from build123d import *

# Parameters (mm, degrees)
BOSS_EXTRUDE1_DEPTH = 9
SKETCH2_R           = 2.875
BOSS_EXTRUDE2_DEPTH = 7
SKETCH3_W           = 1.5
SKETCH3_H           = 1.5
BOSS_EXTRUDE3_DEPTH = 6


with BuildPart() as part:
    # Sketch1 → Boss-Extrude1 (new body)
    with BuildSketch(Plane.XY):
        Polygon((3.4, 0), (1.7, 2.944486373), (-1.7, 2.944486373), (-3.4, 0), (-1.7, -2.944486373), (1.7, -2.944486373), align=None)
    extrude(amount=BOSS_EXTRUDE1_DEPTH)

    # Sketch2 → Boss-Extrude2 (add)
    with BuildSketch(Plane.XY.offset(9)):
        Circle(SKETCH2_R)
    extrude(amount=BOSS_EXTRUDE2_DEPTH)

    # Sketch3 → Boss-Extrude3 (add)
    with BuildSketch(Plane.XY.offset(16)):
        with Locations((0, 2.875)):
            Rectangle(SKETCH3_W, SKETCH3_H)
    extrude(amount=-BOSS_EXTRUDE3_DEPTH)


solid = part.part
Geometry: final body of the model. Coordinates: model frame, mm. A direction names the side the tool comes from. Round coordinates to 2 decimals unless told otherwise and drop trailing zeros. Loops run counter-clockwise (first coordinate to the right, second up) from the corner with the lowest first, then second, coordinate; pieces in that order, holes last.
Q1. Section D-D on y = -2. Return loops of the section in (x, z), plus the area to 3 significant figures.
Q2. Material intervals for L1, parallel to Z at x = 2, y = 2.25; L2, parallel to Y at x = -1.25, z = 6.75; L3, parallel to X at y = -2, z = 13.75, sorted ascending.
Q3. Section B-B on z = 2. Return loops of the section in (x, y).
Q4. Pin query (flat end, axial travel): P1, Ø1.5, axis at x = -0.5, z = 2, coming from the +Y side; P2, Ø2, axis at x = -1, z = 11.5, coming from the -Y side (3 decimals). Return the tip coordinate at first contact, or that it passes through.
Q5. Access query for faces 1 (the flat face through (0.75, 3, 13)), 2 (the flat face through (0, 2.944, 4)), 3 (the flat face through (-0.75, 3, 13)). Directions: +Z, -Z, +X, -X, +Y, -Y. A direction counts if a zero-diameter tool reaches every point of the face in a straight line with its end or side. Return the directions, or none.
Q6. Section A-A on x = 0. Return loops of the section in (y, z) (3 decimals).
Q7. Section C-C on y = 1.5. Return loops of the section in (x, z).
Evaluation:
1. outline: (-2.25, 0) - (2.25, 0) - (2.25, 9) - (2.07, 9) - (2.07, 16) - (-2.07, 16) - (-2.07, 9) - (-2.25, 9) - close
1. area: 69.3 mm2
2. L1: z = 0 to 9
2. L2: y = -2.94 to 2.94
2. L3: x = -2.07 to 2.07
3. outline: (-3.4, 0) - (-1.7, -2.94) - (1.7, -2.94) - (3.4, 0) - (1.7, 2.94) - (-1.7, 2.94) - close
4. P1: stops at y = 2.94
4. P2: stops at y = -2.875
5. face 1: +Z, +X, +Y
5. face 2: -Z, +X, -X, +Y
5. face 3: +Z, -X, +Y
6. outline: (-2.944, 0) - (2.944, 0) - (2.944, 9) - (2.875, 9) - (2.875, 10) - (3.625, 10) - (3.625, 16) - (-2.875, 16) - (-2.875, 9) - (-2.944, 9) - close
7. outline: (-2.53, 0) - (2.53, 0) - (2.53, 9) - (2.45, 9) - (2.45, 16) - (-2.45, 16) - (-2.45, 9) - (-2.53, 9) - close
